```python
from build123d import *

# Parameters (mm, degrees)
SKETCH1_W           = 210
SKETCH1_H           = 34
BOSS_EXTRUDE1_DEPTH = 1
SKETCH2_W           = 210
SKETCH2_H           = 1
BOSS_EXTRUDE2_DEPTH = 9
SKETCH3_W           = 210
SKETCH3_H           = 16
BOSS_EXTRUDE3_DEPTH = 2
FILLET1_R           = 1
FILLET2_R           = 1
FILLET3_R           = 1
FILLET4_R           = 1
FILLET5_R           = 1
FILLET6_R           = 1
CUT_EXTRUDE1_DEPTH  = 211.924156985
FILLET7_R           = 1
FILLET8_R           = 1
FILLET9_R           = 1
FILLET10_R          = 1
SKETCH5_W           = 3
SKETCH5_H           = 3
BOSS_EXTRUDE4_DEPTH = 210
FILLET11_R          = 1
FILLET12_R          = 1
FILLET13_R          = 1
FILLET14_R          = 1
FILLET15_R          = 1
FILLET16_R          = 1
FILLET17_R          = 1
FILLET18_R          = 1
SKETCH6_W           = 1
SKETCH6_H           = 3
CUT_EXTRUDE2_DEPTH  = 210
SKETCH7_R           = 3
CUT_EXTRUDE3_DEPTH  = 10


with BuildPart() as part:
    # Sketch1 → Boss-Extrude1 (new body)
    with BuildSketch(Plane(origin=(0, 0, 0), x_dir=(1, 0, 0), z_dir=(0, 1, 0))):
        Rectangle(SKETCH1_W, SKETCH1_H)
    extrude(amount=BOSS_EXTRUDE1_DEPTH)

    # Sketch2 → Boss-Extrude2 (add)
    with BuildSketch(Plane(origin=(0, 1, 0), x_dir=(1, 0, 0), z_dir=(0, 1, 0))):
        with Locations((0, 16.5)):
            Rectangle(SKETCH2_W, SKETCH2_H)
        with Locations((0, -16.5)):
            Rectangle(SKETCH2_W, SKETCH2_H)
    extrude(amount=BOSS_EXTRUDE2_DEPTH)

    # Sketch3 → Boss-Extrude3 (add)
    with BuildSketch(Plane(origin=(0, 1, 0), x_dir=(1, 0, 0), z_dir=(0, 1, 0))):
        Rectangle(SKETCH3_W, SKETCH3_H)
    extrude(amount=BOSS_EXTRUDE3_DEPTH)

    # Fillet1
    fillet1_edges = [part.edges().sort_by_distance(p)[0] for p in [
        (0, 1, 8),
    ]]
    fillet(fillet1_edges, radius=FILLET1_R)

    # Fillet2
    fillet2_edges = [part.edges().sort_by_distance(p)[0] for p in [
        (0, 1, -8),
    ]]
    fillet(fillet2_edges, radius=FILLET2_R)

    # Fillet3
    fillet3_edges = [part.edges().sort_by_distance(p)[0] for p in [
        (0, 1, 16),
    ]]
    fillet(fillet3_edges, radius=FILLET3_R)

    # Fillet4
    fillet4_edges = [part.edges().sort_by_distance(p)[0] for p in [
        (0, 1, -16),
    ]]
    fillet(fillet4_edges, radius=FILLET4_R)

    # Fillet5
    fillet5_edges = [part.edges().sort_by_distance(p)[0] for p in [
        (0, 10, -16),
    ]]
    fillet(fillet5_edges, radius=FILLET5_R - 0.0001)  # a hair under: the kernel refuses the full size

    # Fillet6
    fillet6_edges = [part.edges().sort_by_distance(p)[0] for p in [
        (0, 10, 16),
    ]]
    fillet(fillet6_edges, radius=FILLET6_R - 0.0001)  # a hair under: the kernel refuses the full size

    # Sketch4 → Cut-Extrude1 (cut, through all)
    with BuildSketch(Plane(origin=(105, 0, 0), x_dir=(0, 0, -1), z_dir=(1, 0, 0))):
        with BuildLine():
            Line((-9, 0), (9, 0))
            ThreePointArc((9, 0), (7.845299462, 0.367006838), (7.114381917, 1.333333333))
            ThreePointArc((7.114381917, 1.333333333), (6.748923144, 1.816496581), (6.171572875, 2))
            Line((6.171572875, 2), (-6.171572875, 2))
            ThreePointArc((-6.171572875, 2), (-6.748923144, 1.816496581), (-7.114381917, 1.333333333))
            ThreePointArc((-7.114381917, 1.333333333), (-7.845299462, 0.367006838), (-9, 0))
        make_face()
    extrude(amount=-CUT_EXTRUDE1_DEPTH, mode=Mode.SUBTRACT)

    # Fillet7
    fillet7_edges = [part.edges().sort_by_distance(p)[0] for p in [
        (0, 3, 8),
    ]]
    fillet(fillet7_edges, radius=FILLET7_R - 0.0001)  # a hair under: the kernel refuses the full size

    # Fillet8
    fillet8_edges = [part.edges().sort_by_distance(p)[0] for p in [
        (0, 3, -8),
    ]]
    fillet(fillet8_edges, radius=FILLET8_R - 0.0001)  # a hair under: the kernel refuses the full size

    # Fillet9
    fillet9_edges = [part.edges().sort_by_distance(p)[0] for p in [
        (0, 0, -17),
    ]]
    fillet(fillet9_edges, radius=FILLET9_R)

    # Fillet10
    fillet10_edges = [part.edges().sort_by_distance(p)[0] for p in [
        (0, 0, 17),
    ]]
    fillet(fillet10_edges, radius=FILLET10_R)

    # Sketch5 → Boss-Extrude4 (add)
    with BuildSketch(Plane(origin=(105, 0, 0), x_dir=(0, 0, -1), z_dir=(1, 0, 0))):
        with Locations((-16.5, 5.371770908)):
            Rectangle(SKETCH5_W, SKETCH5_H)
        with Locations((16.5, 5.371770908)):
            Rectangle(SKETCH5_W, SKETCH5_H)
    extrude(amount=-BOSS_EXTRUDE4_DEPTH)

    # Fillet11
    fillet11_edges = [part.edges().sort_by_distance(p)[0] for p in [
        (0, 6.871770908, 16),
    ]]
    fillet(fillet11_edges, radius=FILLET11_R - 0.0001)  # a hair under: the kernel refuses the full size

    # Fillet12
    fillet12_edges = [part.edges().sort_by_distance(p)[0] for p in [
        (0, 6.871770908, 15),
    ]]
    fillet(fillet12_edges, radius=FILLET12_R)

    # Fillet13
    fillet13_edges = [part.edges().sort_by_distance(p)[0] for p in [
        (0, 3.871770908, 15),
    ]]
    fillet(fillet13_edges, radius=FILLET13_R - 0.0001)  # a hair under: the kernel refuses the full size

    # Fillet14
    fillet14_edges = [part.edges().sort_by_distance(p)[0] for p in [
        (0, 3.871770908, 16),
    ]]
    fillet(fillet14_edges, radius=FILLET14_R)

    # Fillet15
    fillet15_edges = [part.edges().sort_by_distance(p)[0] for p in [
        (0, 6.871770908, -16),
    ]]
    fillet(fillet15_edges, radius=FILLET15_R - 0.0001)  # a hair under: the kernel refuses the full size

    # Fillet16
    fillet16_edges = [part.edges().sort_by_distance(p)[0] for p in [
        (0, 6.871770908, -15),
    ]]
    fillet(fillet16_edges, radius=FILLET16_R)

    # Fillet17
    fillet17_edges = [part.edges().sort_by_distance(p)[0] for p in [
        (0, 3.871770908, -15),
    ]]
    fillet(fillet17_edges, radius=FILLET17_R - 0.0001)  # a hair under: the kernel refuses the full size

    # Fillet18
    fillet18_edges = [part.edges().sort_by_distance(p)[0] for p in [
        (0, 3.871770908, -16),
    ]]
    fillet(fillet18_edges, radius=FILLET18_R)

    # Sketch6 → Cut-Extrude2 (cut)
    with BuildSketch(Plane(origin=(105, 0, 0), x_dir=(0, 0, -1), z_dir=(1, 0, 0))):
        with Locations((-17.5, 5.371770908)):
            Rectangle(SKETCH6_W, SKETCH6_H)
        with Locations((17.5, 5.371770908)):
            Rectangle(SKETCH6_W, SKETCH6_H)
    extrude(amount=-CUT_EXTRUDE2_DEPTH, mode=Mode.SUBTRACT)

    # Sketch7 → Cut-Extrude3 (cut)
    with BuildSketch(Plane.XZ.offset(-2)):
        with Locations(Location((-90, 0, 0), (0, 0, 270))):
            Circle(SKETCH7_R)
    extrude(amount=-CUT_EXTRUDE3_DEPTH, mode=Mode.SUBTRACT)


solid = part.part
```
Design review of the part built by this model. Coordinates are the model's own, in mm. A direction names the side the tool comes from. Give positions to 0.01 mm unless a question says otherwise; leave off trailing zeros. Loops run counter-clockwise (first coordinate to the right, second up) from the corner with the lowest first, then second, coordinate; pieces in that order, holes last. Notation, with made-up numbers: M 43,57.5 L 76,57.5 A20 cw 76,63.5 Z; hole C -25.75,27 d8. An arc over 180 degrees is marked long. Return JSON: item names as keys, results as strings. Group by question number.
Item 1: Mouldability with a two-part tool opening along Z and no side actions: class faces 1 (the flat face through (-105, 2.8, 0.1)), 2 (the flat face through (-1, 1, -12)), 3 (the flat face through (-1, 5, -17)) as released by +Z, released by -Z, zero draft, split by the parting line, or undercut.
Item 2: For probe 1 along Z at (x, y) = (45.5, 7.75); probe 2 along Z at (x, y) = (29, 6); probe 3 along Z at (x, y) = (-59, 1.75), list the stretches that pass through material, from the lowest coordinate up.
Item 3: We need section A-A (z = 0). Give the boundary of the cut face in (x, y).
Item 4: Insertion check: pin 1 Ø3.5 at (x, z) = (11.5, 1.5) entering from -Y; pin 2 Ø3 at (x, z) = (-9, -11) entering from +Y; pin 3 Ø2 at (x, z) = (-68, -0.5) entering from +Y; pin 4 Ø1 at (y, z) = (3, 10) entering from +X. Each pin has a flat end and moves straight along its axis. Give the tip position at first contact, or say it passes through.
Item 5: Tool access review of faces 4 (the cylindrical face through (-92.93, 2.49, 0.65)), 5 (the flat face through (1, 2, 0)), 6 (the flat face through (-1, 1, 12)): name each direction out of +Z, -Z, +X, -X, +Y, -Y from which nothing blocks a thin tool from reaching the whole face with its end or side.
Output:
{
 "1": {"face 1": "zero draft", "face 2": "undercut", "face 3": "released by -Z"},
 "2": {"probe 1": "z = -17 to -15.99, 15.99 to 17", "probe 2": "z = -17 to -15, 15 to 17", "probe 3": "z = -17 to -15.97, -8.03 to -6.83, 6.83 to 8.03, 15.97 to 17"},
 "3": {"outline": "M -105,2 L -93,2 L -93,3 L -105,3 Z; M -87,2 L 105,2 L 105,3 L -87,3 Z"},
 "4": {"pin 1": "stops at y = 2", "pin 2": "stops at y = 1", "pin 3": "stops at y = 3", "pin 4": "passes through"},
 "5": {"face 4": "+Y, -Y", "face 5": "+X, -X, -Y", "face 6": "+X, -X, +Y"}
}
